```python
from build123d import *

# Parameters (mm, degrees)
ESBO_O1_W                  = 114.3
ESBO_O1_H                  = 101.6
RESSALTO_EXTRUS_O1_DEPTH   = 6.35
ESBO_O3_W                  = 74.6252
ESBO_O3_H                  = 89.6874
RESSALTO_EXTRUS_O2_DEPTH   = 129.54
CORTE_EXTRUS_O1_DEPTH      = 129.54
CORTE_EXTRUS_O2_DEPTH      = 17.78
CORTE_EXTRUS_O3_DEPTH      = 17.78
ESBO_O7_R                  = 9.525
CORTE_EXTRUS_O4_DEPTH      = 5.5626
ESBO_O8_R                  = 9.525
CORTE_EXTRUS_O5_DEPTH      = 5.5626
CORTE_EXTRUS_O6_DEPTH      = 31.75
CORTE_EXTRUS_O6_DEPTH_BACK = 31.75


with BuildPart() as part:
    # Esboço1 → Ressalto-extrusão1 (new body)
    with BuildSketch(Plane(origin=(0, 0, 0), x_dir=(1, 0, 0), z_dir=(0, 1, 0))):
        with Locations((57.15, 0)):
            Rectangle(ESBO_O1_W, ESBO_O1_H)
        with BuildLine():
            Line((92.799713965, 34.016189941), (100.737213965, 29.253689941))
            ThreePointArc((100.737213965, 29.253689941), (107.271310059, 30.887213965), (105.637786035, 37.421310059))
            Line((105.637786035, 37.421310059), (97.700286035, 42.183810059))
            ThreePointArc((97.700286035, 42.183810059), (91.166189941, 40.550286035), (92.799713965, 34.016189941))
        make_face(mode=Mode.SUBTRACT)
        with BuildLine():
            Line((97.700286035, -42.183810059), (105.637786035, -37.421310059))
            ThreePointArc((105.637786035, -37.421310059), (107.271310059, -30.887213965), (100.737213965, -29.253689941))
            Line((100.737213965, -29.253689941), (92.799713965, -34.016189941))
            ThreePointArc((92.799713965, -34.016189941), (91.166189941, -40.550286035), (97.700286035, -42.183810059))
        make_face(mode=Mode.SUBTRACT)
        with BuildLine():
            Line((13.562786035, 29.253689941), (21.500286035, 34.016189941))
            ThreePointArc((21.500286035, 34.016189941), (23.133810059, 40.550286035), (16.599713965, 42.183810059))
            Line((16.599713965, 42.183810059), (8.662213965, 37.421310059))
            ThreePointArc((8.662213965, 37.421310059), (7.028689941, 30.887213965), (13.562786035, 29.253689941))
        make_face(mode=Mode.SUBTRACT)
        with BuildLine():
            Line((8.662213965, -37.421310059), (16.599713965, -42.183810059))
            ThreePointArc((16.599713965, -42.183810059), (23.133810059, -40.550286035), (21.500286035, -34.016189941))
            Line((21.500286035, -34.016189941), (13.562786035, -29.253689941))
            ThreePointArc((13.562786035, -29.253689941), (7.028689941, -30.887213965), (8.662213965, -37.421310059))
        make_face(mode=Mode.SUBTRACT)
    extrude(amount=RESSALTO_EXTRUS_O1_DEPTH)

    # Esboço2 → Revolução1 (revolve)
    with BuildSketch(Plane.XY):
        with BuildLine():
            Line((57.15, 0), (96.212075536, 0))
            ThreePointArc((96.212075536, 0), (97.965508733, -5.977876228), (98.425, -12.190637285))
            Line((98.425, -12.190637285), (57.15, -12.190637285))
            Line((57.15, -12.190637285), (57.15, 0))
        make_face()
    revolve(axis=Axis((57.15, -12.190637285, 0), (0, 1, 0)))

    # Esboço3 → Ressalto-extrusão2 (add)
    with BuildSketch(Plane(origin=(0, 0, 0), x_dir=(0, 0, -1), z_dir=(1, 0, 0))):
        with Locations((0, -56.7563)):
            Rectangle(ESBO_O3_W, ESBO_O3_H)
    extrude(amount=RESSALTO_EXTRUS_O2_DEPTH)

    # Esboço4 → Corte-extrusão1 (cut)
    with BuildSketch(Plane(origin=(0, 0, 0), x_dir=(0, 0, -1), z_dir=(1, 0, 0))):
        with BuildLine():
            Line((-31.75, -27.323981416), (-31.75, -101.6))
            Line((-31.75, -101.6), (31.75, -101.6))
            Line((31.75, -101.6), (31.75, -27.323981416))
            ThreePointArc((31.75, -27.323981416), (28.496991957, -17.652408672), (20.060406327, -11.9126))
            Line((20.060406327, -11.9126), (-20.060406327, -11.9126))
            ThreePointArc((-20.060406327, -11.9126), (-28.496991957, -17.652408672), (-31.75, -27.323981416))
        make_face()
    extrude(amount=CORTE_EXTRUS_O1_DEPTH, mode=Mode.SUBTRACT)

    # Esboço5 → Corte-extrusão2 (cut)
    with BuildSketch(Plane.XY.offset(37.3126)):
        with BuildLine():
            Line((0, -11.9126), (0, -113.5126))
            Line((0, -113.5126), (129.54, -113.5126))
            Line((129.54, -113.5126), (129.54, -11.9126))
            Line((129.54, -11.9126), (94.472692749, -11.9126))
            Line((94.472692749, -11.9126), (94.472692749, -25.121962715))
            Line((94.472692749, -25.121962715), (122.05004704, -78.430872329))
            ThreePointArc((122.05004704, -78.430872329), (116.924107122, -98.820076417), (96.059025593, -96.242621055))
            Line((96.059025593, -96.242621055), (41.979486254, -35.10156883))
            ThreePointArc((41.979486254, -35.10156883), (35.071399527, -28.539398345), (26.177307251, -25.121962715))
            Line((26.177307251, -25.121962715), (19.827307251, -25.121962715))
            Line((19.827307251, -25.121962715), (19.827307251, -11.9126))
            Line((19.827307251, -11.9126), (0, -11.9126))
        make_face()
    extrude(amount=-CORTE_EXTRUS_O2_DEPTH, mode=Mode.SUBTRACT)

    # Esboço6 → Corte-extrusão3 (cut)
    with BuildSketch(Plane.XY.offset(-37.3126)):
        with BuildLine():
            Line((0, -11.9126), (0, -113.5126))
            Line((0, -113.5126), (129.54, -113.5126))
            Line((129.54, -113.5126), (129.54, -11.9126))
            Line((129.54, -11.9126), (94.472692749, -11.9126))
            Line((94.472692749, -11.9126), (94.472692749, -25.121962715))
            Line((94.472692749, -25.121962715), (122.05004704, -78.430872329))
            ThreePointArc((122.05004704, -78.430872329), (116.924107122, -98.820076417), (96.059025593, -96.242621055))
            Line((96.059025593, -96.242621055), (41.979486254, -35.10156883))
            ThreePointArc((41.979486254, -35.10156883), (35.071399527, -28.539398345), (26.177307251, -25.121962715))
            Line((26.177307251, -25.121962715), (19.827307251, -25.121962715))
            Line((19.827307251, -25.121962715), (19.827307251, -11.9126))
            Line((19.827307251, -11.9126), (0, -11.9126))
        make_face()
    extrude(amount=CORTE_EXTRUS_O3_DEPTH, mode=Mode.SUBTRACT)

    # Esboço7 → Corte-extrusão4 (cut)
    with BuildSketch(Plane.XY.offset(37.3126)):
        with Locations((107.95, -85.725)):
            Circle(ESBO_O7_R)
    extrude(amount=-CORTE_EXTRUS_O4_DEPTH, mode=Mode.SUBTRACT)

    # Esboço8 → Corte-extrusão5 (cut)
    with BuildSketch(Plane.XY.offset(-37.3126)):
        with Locations((107.95, -85.725)):
            Circle(ESBO_O8_R)
    extrude(amount=CORTE_EXTRUS_O5_DEPTH, mode=Mode.SUBTRACT)

    # Esboço9 → Corte-extrusão6 (cut, two sides)
    with BuildSketch(Plane.XY) as corte_extrus_o6_sk:
        with BuildLine():
            Line((79.375, -65.0875), (150.000604013, -65.0875))
            ThreePointArc((150.000604013, -65.0875), (166.323156329, -59.148596729), (175.012790586, -44.109097315))
            Line((175.012790586, -44.109097315), (110.495145555, -17.4625))
            Line((110.495145555, -17.4625), (79.375, -17.4625))
            ThreePointArc((79.375, -17.4625), (72.639807909, -20.252307909), (69.85, -26.9875))
            Line((69.85, -26.9875), (69.85, -55.5625))
            ThreePointArc((69.85, -55.5625), (72.639807909, -62.297692091), (79.375, -65.0875))
        make_face()
    extrude(amount=CORTE_EXTRUS_O6_DEPTH, mode=Mode.SUBTRACT)
    extrude(corte_extrus_o6_sk.sketch, amount=-CORTE_EXTRUS_O6_DEPTH_BACK, mode=Mode.SUBTRACT)


solid = part.part
```
Could you check a few things on this model? Use its own coordinates, in mm. A direction names the side the tool comes from. Coordinates: 2 decimals unless noted, no trailing zeros. Order: outer loops, then holes, each group sorted by start corner. A loop starts at its lowest first (then second) coordinate and runs counter-clockwise, first axis right, second up. Notation, with made-up numbers: M 45.25,69.5 L 63.25,69.5 A29 cw 63.25,94.5 Z; hole C 76.5,27 d8. An arc over 180 degrees is marked long. Use a Markdown table: item, result. Add a question column.
Q1. If I drill on L1, parallel to Z at x = 75, y = -63.5; L2, parallel to Y at x = 107.95, z = -35.1; L3, parallel to Z at x = 62, y = -17.5, over which ranges is the centre line in solid material (lowest first)?
Q2. Which directions (+Z, -Z, +X, -X, +Y, -Y) give clear straight access to the entire face, cutting with the end or side of a thin tool? Please do faces 4 (the cylindrical face through (107.324, 3.131, 30.978)), 5 (the cylindrical face through (48.33, -15.82, 26.87)), 6 (the flat face through (87, -17.462, 30)), 7 (the flat face through (23, -25.122, -34)).
Q3. I'm going to push flat-ended pins straight in: pin 1 (1 mm diameter, centred on x = 47.5, z = -37.5, fed in from -Y); pin 2 (10.5 mm diameter, centred on y = -15.5, z = -27.5, fed in from +X); pin 3 (2 mm diameter, centred on x = 64.5, z = 40, fed in from -Y). Where does each tip first touch, or does it pass through?
Q4. I want a section at B-B on y = -14. List the corners of the cut face in (x, z) for me.
Q5. We'd pull the mould along Y, two halves only. Please class faces 1 (the flat face through (25, -11.913, 33)), 2 (the flat face through (83, -47, 37.313)), 3 (the cylindrical face through (117.188, -98.636, 34.57)): pulls with the +Y half, pulls with the -Y half, needs draft (parallel to the pull), parting line crosses it, or undercut.
Q6. I want a section at A-A on y = -74. List the corners of the cut face in (x, z) for me.
Checked values:
| question | item | result |
|---|---|---|
| 1 | L1 | -37.31 to -31.75, 31.75 to 37.31 |
| 1 | L2 | -101.6 to -95.25, -76.2 to -51.17, 0 to 6.35 |
| 1 | L3 | -37.31 to -28.38, 28.38 to 37.31 |
| 2 | face 4 | +Y |
| 2 | face 5 | +X, -X, -Y |
| 2 | face 6 | +X, -Y |
| 2 | face 7 | +Z, -Z, -X, -Y |
| 3 | pin 1 | y = -41.87 |
| 3 | pin 2 | x = 94.47 |
| 3 | pin 3 | y = -12.19 |
| 4 | outline | M 19.83,-37.31 L 94.47,-37.31 L 94.47,-24.61 L 19.83,-24.61 Z; M 19.83,24.61 L 94.47,24.61 L 94.47,37.31 L 19.83,37.31 Z |
| 5 | face 1 | undercut |
| 5 | face 2 | needs draft |
| 5 | face 3 | parting line crosses it |
| 6 | outline | M 76.39,-37.31 L 119.76,-37.31 L 119.76,-31.75 L 76.39,-31.75 Z; M 76.39,31.75 L 119.76,31.75 L 119.76,37.31 L 76.39,37.31 Z |
